Check sheet for the modelled part. Datum: model origin and axes. Units: mm. A direction names the side the tool comes from. Give positions to 0.01 mm unless a question says otherwise; leave off trailing zeros. Loops run counter-clockwise (first coordinate to the right, second up) from the corner with the lowest first, then second, coordinate; pieces in that order, holes last. Notation, with made-up numbers: M 40.5,68 L 65.5,68 A4 cw 65.5,74 Z; hole C 71,1 d9. An arc over 180 degrees is marked long. Use one line per item in the form item = value.
from build123d import *

# Parameters (mm, degrees)
F0_R     = 12.065
F1_DEPTH = 6.35


with BuildPart() as f1:
    # F0 (on Top) → F1 (new body)
    with BuildSketch(Plane.XY):
        Circle(F0_R)
        with BuildLine():
            ThreePointArc((1.190625, 9.27106), (7.017804, 6.174186), (9.3472, 0))
            ThreePointArc((9.3472, 0), (-6.174186, -7.017804), (-1.190625, 9.27106))
            Line((-1.190625, 9.27106), (-1.190625, 10.14095))
            Line((-1.190625, 10.14095), (1.190625, 10.14095))
            Line((1.190625, 10.14095), (1.190625, 9.27106))
        make_face(mode=Mode.SUBTRACT)
    extrude(amount=F1_DEPTH)


solid = f1.part
1) Section check A-A (x = 0). Record the cut outline in (y, z) (3 decimals), then the cut area to 3 significant figures.
Evaluation:
outline = M -12.065,0 L -9.347,0 L -9.347,6.35 L -12.065,6.35 Z; M 10.141,0 L 12.065,0 L 12.065,6.35 L 10.141,6.35 Z
area = 29.5 mm^2
2) Depth check by flat-ended pin: pin 1 Ø1.5 at (x, z) = (9.5, 4) entering from -Y. Enter the tip coordinate at first touch or a pass-through.
Evaluation:
pin_1 = -8.31
3) Release check for a two-part mould opening along Y. For faces 1 (the face through (11.51, 3.62, 3.13)), 2 (the face through (-5.4, -8, 6.35)), 3 (the face through (-1.191, 9.7, 3.1)) record: pulls with the +Y half, pulls with the -Y half, needs draft (parallel to the pull), parting line crosses it, or undercut.
Evaluation:
face_1 = parting line crosses it
face_2 = needs draft
face_3 = undercut
4) Section check C-C (z = 5). Record the cut outline in (x, y) (3 decimals), then the cut area to 3 significant figures.
Evaluation:
outline = C 0,0 d24.13; hole M -1.191,9.271 A9.347 ccw long 1.191,9.271 L 1.191,10.141 L -1.191,10.141 Z
area = 181 mm^2
5) Set-up check for faces 4 (the face through (-5.4, -8, 0)), 5 (the face through (1.191, 9.7, 3.1)): record each of +Z, -Z, +X, -X, +Y, -Y from which the full face is reachable in a straight line by a thin tool's end or side.
Evaluation:
face_4 = -Z, +X, -X, +Y, -Y
face_5 = +Z, -Z
6) Scan lines: line 1 (Y direction, x = 0, z = 3) (3 decimals); line 2 (Y direction, x = -6.25, z = 3.5); line 3 (X direction, y = 5.5, z = 3). Record each from-to range of solid material in increasing order.
Evaluation:
line_1 = -12.065 to -9.347, 10.141 to 12.065
line_2 = -10.32 to -6.95, 6.95 to 10.32
line_3 = -10.74 to -7.56, 7.56 to 10.74
7) Section check B-B (y = -7.5). Record the cut outline in (x, z), then the cut area to 3 significant figures.
Evaluation:
outline = M -9.45,0 L -5.58,0 L -5.58,6.35 L -9.45,6.35 Z; M 5.58,0 L 9.45,0 L 9.45,6.35 L 5.58,6.35 Z
area = 49.2 mm^2
